Work out the finished part from the listing and answer in its coordinate system (mm). A direction names the side the tool comes from. Round coordinates to 2 decimals unless told otherwise and drop trailing zeros. Order: outer loops, then holes, each group sorted by start corner. A loop starts at its lowest first (then second) coordinate and runs counter-clockwise, first axis right, second up. Notation, with made-up numbers: (22.25, -4) - (45.25, -4) arc R37 cw to (45.25, 32) - close; hole circle Ø1 at (86, 89.5). An arc over 180 degrees is marked (long way). Answer in a Markdown table with one row per item.
from build123d import *

# Parameters (mm, degrees)
SKETCH1_R           = 40.3
BOSS_EXTRUDE1_DEPTH = 5
SKETCH2_W           = 40.2
SKETCH2_H           = 20.2
CUT_EXTRUDE3_DEPTH  = 1
SKETCH3_R           = 1.5
CUT_EXTRUDE4_DEPTH  = 6
CUT_EXTRUDE5_REACH  = 7
SKETCH4_R           = 1.5
SKETCH5_R           = 1.5
CUT_EXTRUDE6_DEPTH  = 6


with BuildPart() as part:
    # Sketch1 → Boss-Extrude1 (new body)
    with BuildSketch(Plane(origin=(0, 0, 0), x_dir=(1, 0, 0), z_dir=(0, 1, 0))):
        Circle(SKETCH1_R)
    extrude(amount=BOSS_EXTRUDE1_DEPTH)

    # Sketch2 → Cut-Extrude3 (cut)
    with BuildSketch(Plane(origin=(0, 5, 0), x_dir=(1, 0, 0), z_dir=(0, 1, 0))):
        with Locations((9.6, 0)):
            Rectangle(SKETCH2_W, SKETCH2_H)
    extrude(amount=-CUT_EXTRUDE3_DEPTH, mode=Mode.SUBTRACT)

    # Sketch3 → Cut-Extrude4 (cut, through all)
    with BuildSketch(Plane(origin=(0, 5, 0), x_dir=(1, 0, 0), z_dir=(0, 1, 0))):
        with Locations((-17, -6)):
            Circle(SKETCH3_R)
        with Locations((-17, 0)):
            Circle(SKETCH3_R)
        with Locations((-17, 6)):
            Circle(SKETCH3_R)
        with Locations((36.2, -6)):
            Circle(SKETCH3_R)
        with Locations((36.2, 0)):
            Circle(SKETCH3_R)
        with Locations((36.2, 6)):
            Circle(SKETCH3_R)
    extrude(amount=-CUT_EXTRUDE4_DEPTH, mode=Mode.SUBTRACT)

    # Sketch4 → Cut-Extrude5 (cut, up to next)
    with BuildSketch(Plane(origin=(0, 5, 0), x_dir=(1, 0, 0), z_dir=(0, 1, 0)), mode=Mode.PRIVATE) as cut_extrude5_sk1:
        with Locations((-32.113081447, 5)):
            Circle(SKETCH4_R)
    cut_extrude5_tool1 = extrude(cut_extrude5_sk1.sketch, amount=-CUT_EXTRUDE5_REACH, mode=Mode.PRIVATE) & part.part
    add(cut_extrude5_tool1.solids().sort_by_distance((-32.113081, 5, -5))[0], mode=Mode.SUBTRACT)
    # Sketch4 → Cut-Extrude5 (cut, up to next)
    with BuildSketch(Plane(origin=(0, 5, 0), x_dir=(1, 0, 0), z_dir=(0, 1, 0)), mode=Mode.PRIVATE) as cut_extrude5_sk2:
        with Locations((-32.113081447, -5)):
            Circle(SKETCH4_R)
    cut_extrude5_tool2 = extrude(cut_extrude5_sk2.sketch, amount=-CUT_EXTRUDE5_REACH, mode=Mode.PRIVATE) & part.part
    add(cut_extrude5_tool2.solids().sort_by_distance((-32.113081, 5, 5))[0], mode=Mode.SUBTRACT)

    # Sketch5 → Cut-Extrude6 (cut, through all)
    with BuildSketch(Plane(origin=(0, 5, 0), x_dir=(1, 0, 0), z_dir=(0, 1, 0))):
        with Locations((-32.113081447, 5)):
            Circle(SKETCH5_R)
        with Locations((-32.113081447, -5)):
            Circle(SKETCH5_R)
        with Locations((-21.386109545, 24.472113078)):
            Circle(SKETCH5_R)
        with Locations((-27.813985642, 16.811668647)):
            Circle(SKETCH5_R)
        with Locations((-0.652339307, 32.49345247)):
            Circle(SKETCH5_R)
        with Locations((-10.500416838, 30.756970693)):
            Circle(SKETCH5_R)
        with Locations((20.386667742, 25.310744327)):
            Circle(SKETCH5_R)
        with Locations((11.726413704, 30.310744327)):
            Circle(SKETCH5_R)
        with Locations((-27.813985642, -16.811668647)):
            Circle(SKETCH5_R)
        with Locations((-21.386109545, -24.472113078)):
            Circle(SKETCH5_R)
        with Locations((-10.500416838, -30.756970693)):
            Circle(SKETCH5_R)
        with Locations((-0.652339307, -32.49345247)):
            Circle(SKETCH5_R)
        with Locations((11.726413704, -30.310744327)):
            Circle(SKETCH5_R)
        with Locations((20.386667742, -25.310744327)):
            Circle(SKETCH5_R)
    extrude(amount=-CUT_EXTRUDE6_DEPTH, mode=Mode.SUBTRACT)


solid = part.part
1) Each of these flat-tipped pins is pushed along its axis until it touches: pin 1 (8 mm diameter, centred on x = 3, z = -2.5, fed in from +Y); pin 2 (2.5 mm diameter, centred on x = -21.39, z = 24.47, fed in from +Y); pin 3 (0.5 mm diameter, centred on x = 4.5, y = 4.5, fed in from +Z); pin 4 (1 mm diameter, centred on x = 27.5, y = 3.5, fed in from -Z). Where does it stop, or does it pass through?
Filled in:
| item | result |
|---|---|
| pin 1 | stops at y = 4 |
| pin 2 | passes through |
| pin 3 | stops at z = 40.08 |
| pin 4 | stops at z = -29.92 |
2) Find section B-B, the plane x = 36.2. Give the vertices of the cut face in (y, z).
Filled in:
| item | result |
|---|---|
| outline | (0, -17.71) - (5, -17.71) - (5, -7.5) - (0, -7.5) - close; (0, -4.5) - (5, -4.5) - (5, -1.5) - (0, -1.5) - close; (0, 1.5) - (5, 1.5) - (5, 4.5) - (0, 4.5) - close; (0, 7.5) - (5, 7.5) - (5, 17.71) - (0, 17.71) - close |
3) Find section C-C, the plane y = 1.1. Give the number of separate pieces and of enclosed holes in the cut face, then the cut area to 3 significant figures.
Filled in:
| item | result |
|---|---|
| separate pieces | 1 |
| enclosed holes | 20 |
| area | 4,960 mm^2 |
4) Find the intervals of material crossed by probe 1 along Z at (x, y) = (36.2, 3.55); probe 2 along X at (y, z) = (3.65, 5); probe 3 along Z at (x, y) = (1, 4.3), in increasing order. Write a range as from..to.
Filled in:
| item | result |
|---|---|
| probe 1 | z = -17.71..-7.5, -4.5..-1.5, 1.5..4.5, 7.5..17.71 |
| probe 2 | x = -39.99..-33.61, -30.61..-18.12, -15.88..35.08, 37.32..39.99 |
| probe 3 | z = -40.29..-10.1, 10.1..40.29 |
5) Find section A-A, the plane z = 0. Give the vertices of the cut face in (x, y), then the cut area to 3 significant figures.
Filled in:
| item | result |
|---|---|
| outline | (-40.3, 0) - (-18.5, 0) - (-18.5, 5) - (-40.3, 5) - close; (-15.5, 0) - (34.7, 0) - (34.7, 5) - (29.7, 5) - (29.7, 4) - (-10.5, 4) - (-10.5, 5) - (-15.5, 5) - close; (37.7, 0) - (40.3, 0) - (40.3, 5) - (37.7, 5) - close |
| area | 333 mm^2 |
6) The mould has two halves that part along Z. Classify faces 1 (the face through (35, 2.5, 0.9)), 2 (the face through (-1, 5, 17)), 3 (the face through (37.227, 2.465, 15.435)): released by +Z, released by -Z, zero draft, split by the parting line, or undercut.
Filled in:
| item | result |
|---|---|
| face 1 | undercut |
| face 2 | zero draft |
| face 3 | split by the parting line |
7) Which of the six approach directions +Z, -Z, +X, -X, +Y, -Y give full straight-line access (tool end or side, diameter ignored) to faces 4 (the face through (9, 4, 0)), 5 (the face through (-1, 0, -1))?
Filled in:
| item | result |
|---|---|
| face 4 | +Y |
| face 5 | +Z, -Z, +X, -X, -Y |
8) Find section D-D, the plane x = 27. Give the vertices of the cut face in (y, z).
Filled in:
| item | result |
|---|---|
| outline | (0, -29.92) - (5, -29.92) - (5, -10.1) - (4, -10.1) - (4, 10.1) - (5, 10.1) - (5, 29.92) - (0, 29.92) - close |
